Check sheet for the drawn part. Datum: minimum x, y, z corner. Units: mm. Coordinates: 2 decimals unless noted, no trailing zeros. Order: outer loops, then holes, each group sorted by start corner. A loop starts at its lowest first (then second) coordinate and runs counter-clockwise, first axis right, second up.
Q1. Cross-section at A-A, the plane x = 3. Record the boundary of the cut face in (y, z), and give its area (3 significant figures).
Q2. Cross-section at B-B, the plane z = 7.5. Record the boundary of the cut face in (x, y), and give its area (3 significant figures).
Q3. Depth check by flat-ended pin: P1, Ø2, axis at x = 6.5, y = 25.5, coming from the +Z side. Enter the tip coordinate at first touch or a pass-through.
Q4. Thickness scan on line 1 (X direction, y = 64, z = 5.5); line 2 (X direction, y = 54.5, z = 11.5); line 3 (Z direction, x = 10, y = 14.5). Record the ranges inside material, lowest first.
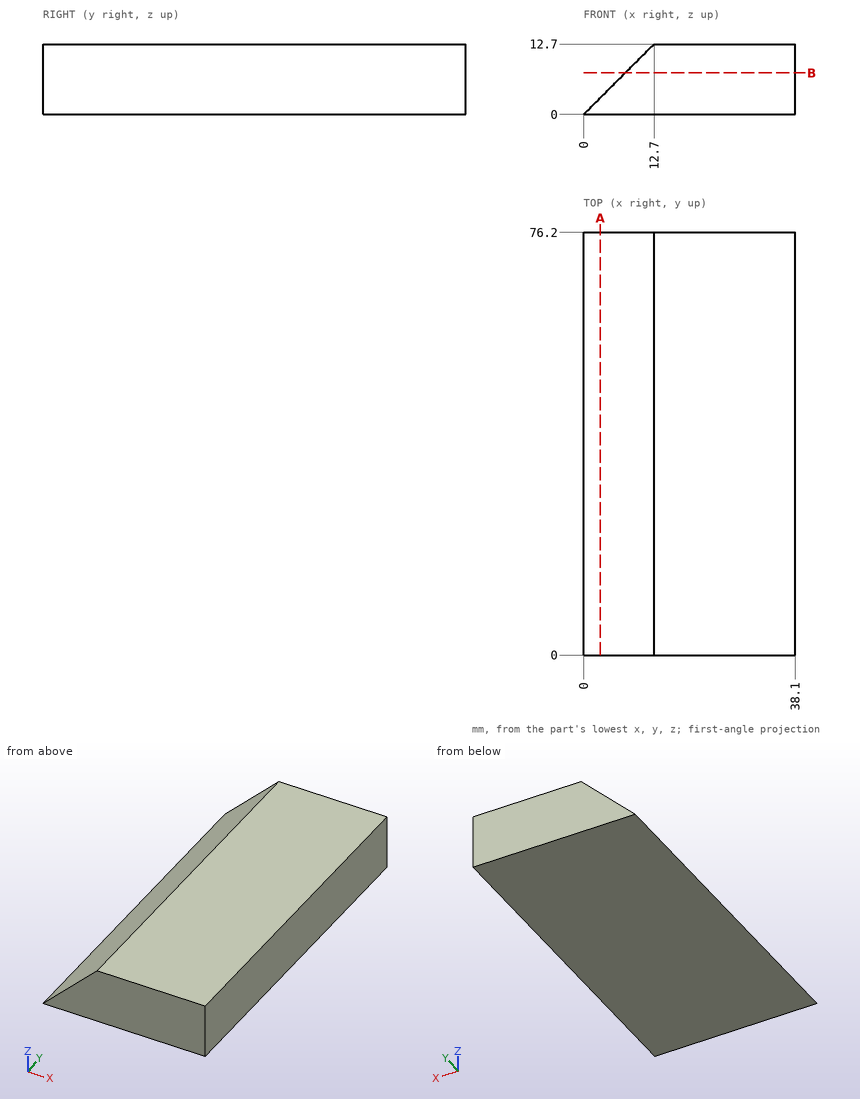
Check values:
1. outline: (0, 0) - (76.2, 0) - (76.2, 3) - (0, 3) - close
1. area: 229 mm2
2. outline: (7.5, 0) - (38.1, 0) - (38.1, 76.2) - (7.5, 76.2) - close
2. area: 2,330 mm2
3. P1: stops at z = 7.5
4. line 1: x = 5.5 to 38.1
4. line 2: x = 11.5 to 38.1
4. line 3: z = 0 to 10
